Print and shaded views of the part. All mm, measured from the part's lowest x, y and z. Coordinates: 2 decimals unless noted, no trailing zeros. Order: outer loops, then holes, each group sorted by start corner. A loop starts at its lowest first (then second) coordinate and runs counter-clockwise, first axis right, second up. Notation, with made-up numbers: (-14, 25.25) -> (38, 25.25) arc R20 ccw to (38, 55.25) -> close; hole circle Ø11 at (-28.5, -39). An arc over 180 degrees is marked (long way). Return JSON: item names as keys, results as strings. Group by question number.
1) Probe line 1 (X direction, y = 5, z = 23.5) (1 decimal); line 2 (X direction, y = 8.75, z = 21.5) (1 decimal); line 3 (Z direction, x = 126, y = 1) (1 decimal). List the from-to ranges inside material, lowest first.
2) Cut at A-A (y = 2). Write the cut outline in (x, z) (1 decimal).
3) Flat gauge pin, fed straight in: pin 1 (10 mm diameter, centred on x = 20.77, z = 23.81, fed in from -Y). Where does the tip first touch, or does it go through?
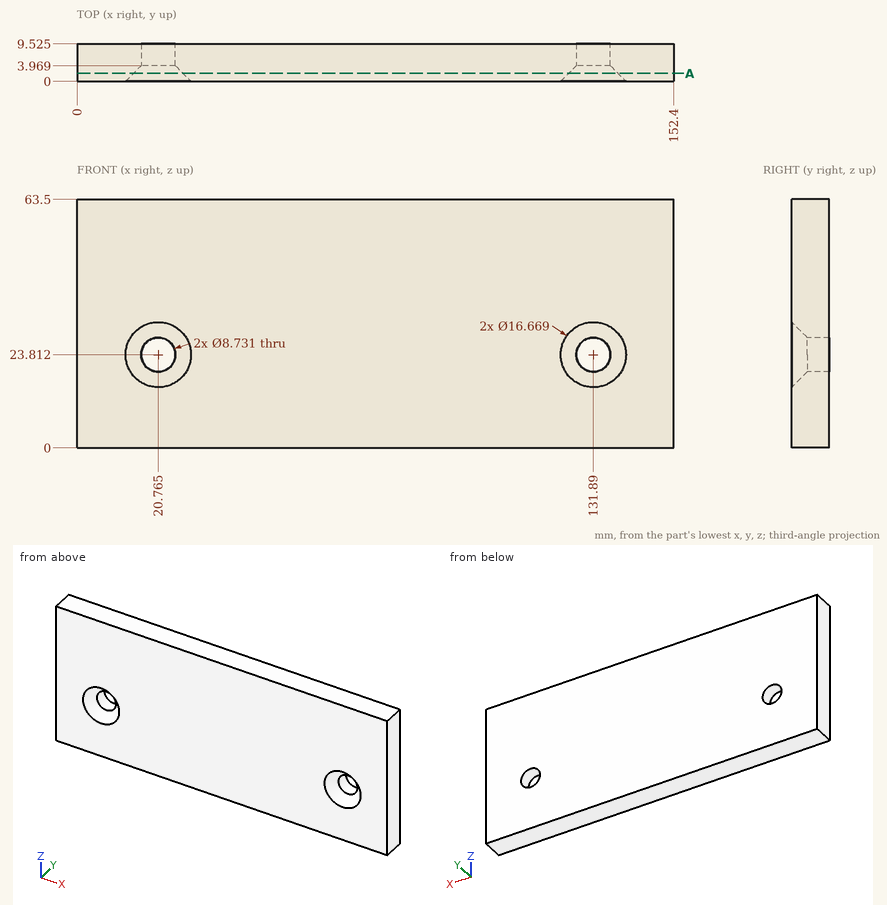
Answers below:
{
 "1": {"line 1": "x = 0 to 16.4, 25.1 to 127.5, 136.2 to 152.4", "line 2": "x = 0 to 17.1, 24.5 to 128.2, 135.6 to 152.4", "line 3": "z = 0 to 19.4, 28.2 to 63.5"},
 "2": {"outline": "(0, 0) -> (152.4, 0) -> (152.4, 63.5) -> (0, 63.5) -> close; hole circle Ø12.7 at (20.8, 23.8); hole circle Ø12.7 at (131.9, 23.8)"},
 "3": {"pin 1": "stops at y = 3.33"}
}
